Autodesk Inventor part; units mm, degrees
ref_plane "YZ Plane" through (0, 0, 0) normal (1, 0, 0) x (0, 1, 0)
ref_plane "XZ Plane" through (0, 0, 0) normal (0, 1, 0) x (-1, 0, 0)
ref_plane "XY Plane" through (0, 0, 0) normal (0, 0, 1) x (1, 0, 0)
sketch "Sketch1" plane through (0, 0, 0) normal (0, 1, 0) x (-1, 0, 0)
  line L0 (-545.8153, 185.3726) -> (-326.5965, 142.7608)
  line L1 (-545.8153, -185.3726) -> (-326.5965, -142.7608)
  arc A0 (-545.8153, -185.3726) -> (-545.8153, 185.3726) centre (0, 0) ccw
  arc A1 (-326.5965, -142.7608) -> (-326.5965, 142.7608) centre (0, 0) ccw
  arc A2 (-324.2, -138.2201) -> (-324.2, 138.2201) centre (0, 0) ccw
  arc A3 (-551.0584, -182.3169) -> (-551.0584, 182.3169) centre (0, 0) ccw
  line L2 (-551.0584, 182.3169) -> (-324.2, 138.2201)
  line L3 (-324.2, -138.2201) -> (-551.0584, -182.3169)
  dimension "d81" = 4
  dimension "d82" = 4
extrude "Extrusion2" add sketch "Sketch1" along normal blind 30
properties part number "Level 2 Edge Banding"
Can you work these out from the model? Positions are in its coordinate system, mm. A direction names the side the tool comes from. Coordinates: 2 decimals unless noted, no trailing zeros. Loops run counter-clockwise (first coordinate to the right, second up) from the corner with the lowest first, then second, coordinate; pieces in that order, holes last. Notation, with made-up numbers: M 3.5,15 L 32.5,15 A18 cw 32.5,29 Z; hole C 85.25,78.5 d6. An arc over 180 degrees is marked long. Return JSON: item names as keys, results as strings. Group by question number.
Item 1: I'm going to push flat-ended pins straight in: pin 1 Ø4 at (x, y) = (-113.5, 9) entering from -Z; pin 2 Ø4 at (x, y) = (158, 25) entering from -Z; pin 3 Ø2 at (x, y) = (-181.5, 7.5) entering from -Z. Where does each tip first touch, or does it pass through?
Item 2: Imagine slicing it at D-D (y = 21.75). Please give me the cut outline in (x, z) (1 decimal), and give its area (3 significant figures).
Item 3: Thinking about a two-plate mould opening in X: for faces 1 (the cylindrical face through (-579.98, 14.79, 22.93)), 2 (the cylindrical face through (-356.175, 14.79, 13.617)), 3 (the flat face through (-180, 0, 304)), which applies, released by +X, released by -X, zero draft, split by the parting line, or undercut?
Item 4: Imagine slicing it at C-C (z = 299.5). Please give me the cut outline in (x, y).
Item 5: Imagine slicing it at A-A (x = 0). Please give me the cut outline in (y, z) (3 decimals), and give its area (3 significant figures).
Item 6: Imagine slicing it at B-B (z = 0). Please give me the cut outline in (x, y) (3 decimals), and give its area (3 significant figures).
Item 7: On a 3-axis mill with a long thin cutter (end or side, diameter ignored), from which of +Z, -Z, +X, -X, +Y, -Y can I reach the whole of each face in a straight line? I mean faces 4 (the flat face through (437.74, 14.79, -164.365)), 5 (the flat face through (-180, 30, 304)), 6 (the flat face through (439.217, 14.79, 160.577)). Say none if no direction works.
Item 8: If I drill on L1, parallel to Z at x = 0, y = 14.5 (3 decimals); L2, parallel to Z at x = 252.5, y = 25; L3, parallel to X at y = 5.75, z = -305.5, over which ranges is the centre line in solid material (lowest first)? Write a range as from..to.
Verdict:
{
 "1": {"pin 1": "stops at z = -569.62", "pin 2": "stops at z = -559.08", "pin 3": "stops at z = -551.66"},
 "2": {"outline": "M 324.2,-138.2 A352.4 cw long 324.2,138.2 L 551.1,182.3 A580.4 ccw long 551.1,-182.3 Z; hole M 326.6,-142.8 A356.4 cw long 326.6,142.8 L 545.8,185.4 A576.4 ccw long 545.8,-185.4 Z", "area": "22,600 mm^2"},
 "3": {"face 1": "split by the parting line", "face 2": "undercut", "face 3": "zero draft"},
 "4": {"outline": "M -497.2,0 L -492.52,0 L -492.52,30 L -497.2,30 Z; M -193.25,0 L -185.77,0 L -185.77,30 L -193.25,30 Z; M 185.77,0 L 193.25,0 L 193.25,30 L 185.77,30 Z; M 492.52,0 L 497.2,0 L 497.2,30 L 492.52,30 Z"},
 "5": {"outline": "M 0,-580.435 L 30,-580.435 L 30,-576.435 L 0,-576.435 Z; M 0,-356.435 L 30,-356.435 L 30,-352.435 L 0,-352.435 Z; M 0,352.435 L 30,352.435 L 30,356.435 L 0,356.435 Z; M 0,576.435 L 30,576.435 L 30,580.435 L 0,580.435 Z", "area": "480 mm^2"},
 "6": {"outline": "M -580.435,0 L -576.435,0 L -576.435,30 L -580.435,30 Z; M -356.435,0 L -352.435,0 L -352.435,30 L -356.435,30 Z", "area": "240 mm^2"},
 "7": {"face 4": "+Y, -Y", "face 5": "+Z, -Z, +X, -X, +Y", "face 6": "+X, +Y, -Y"},
 "8": {"L1": "z = -580.435..-576.435, -356.435..-352.435, 352.435..356.435, 576.435..580.435", "L2": "z = -522.64..-518.19, -251.57..-245.87, 245.87..251.57, 518.19..522.64", "L3": "x = -493.53..-488.82, -183.62..-175.73, 175.73..183.62, 488.82..493.53"}
}
